Job drawing, mm, ordinate dimensions from the low corner. One solid piece. A direction names the side the tool comes from. Round coordinates to 2 decimals unless told otherwise and drop trailing zeros. Loops run counter-clockwise (first coordinate to the right, second up) from the corner with the lowest first, then second, coordinate; pieces in that order, holes last. Notation, with made-up numbers: M -37,40 L -27,40 A27 cw -27,78 Z; hole C 13.5,26 d8. An arc over 180 degrees is marked long. Put each result on its own line as item: value. Start each with the question number.
1) Probe line 1 along X through (y, z) = (1.25, 7); line 2 along X through (y, z) = (10, 5); line 3 along Y through (x, z) = (17, 3) (1 decimal). List the from-to ranges inside material, lowest first.
2) Slice it at A-A on y = 6.5. Give the cut face in (x, z).
3) Which spindle directions (+Z, -Z, +X, -X, +Y, -Y) get a long thin tool onto all of the face, cutting with end or side? Do the marked faces 1 and 2. Say none if no direction does.
4) Drop flat-ended pins along their axis: pin 1 Ø4 at (x, y) = (18.5, 4.5) entering from +Z; pin 2 Ø1.2 at (y, z) = (7, 6) entering from -X; pin 3 Ø5 at (x, z) = (35.5, 9) entering from +Y. Give the stop position or say it passes through.
5) Slice it at B-B on x = 6.5. Give the cut face in (y, z).
6) Pull direction Y, two halves, no side cores. Call the marked faces 3, 4 and 5: +Y half, -Y half, draft (parallel to the pull), parting line (faces both ways), or undercut.
7) Slice it at C-C on x = 52.5. Give the cut face in (y, z), then the cut area to 3 significant figures.
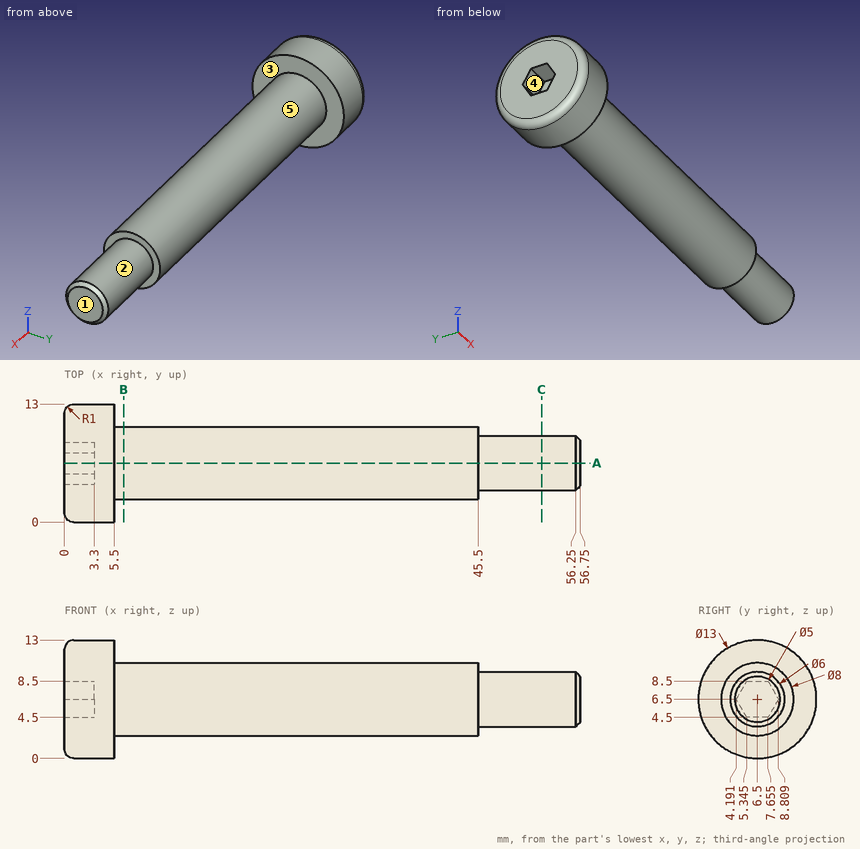
Recorded:
1. line 1: x = 0 to 5.5
1. line 2: x = 0 to 45.5
1. line 3: y = 4.6 to 8.4
2. outline: M 0,1 A1 ccw 1,0 L 5.5,0 L 5.5,2.5 L 45.5,2.5 L 45.5,3.5 L 56.25,3.5 L 56.75,4 L 56.75,9 L 56.25,9.5 L 45.5,9.5 L 45.5,10.5 L 5.5,10.5 L 5.5,13 L 1,13 A1 ccw 0,12 L 0,8.5 L 3.3,8.5 L 3.3,4.5 L 0,4.5 Z
3. face 1: +Z, -Z, +X, +Y, -Y
3. face 2: +X
4. pin 1: stops at z = 10.5
4. pin 2: stops at x = 3.3
4. pin 3: stops at y = 10.5
5. outline: C 6.5,6.5 d8
6. face 3: draft
6. face 4: undercut
6. face 5: parting line
7. outline: C 6.5,6.5 d6
7. area: 28.3 mm2
